```python
from build123d import *

# Parameters (mm, degrees)
SKETCH1_R           = 1.4
BOSS_EXTRUDE1_DEPTH = 19
SKETCH2_R           = 1.7
BOSS_EXTRUDE2_DEPTH = 0.7
FILLET1_R           = 0.5
SKETCH3_R           = 1.7
BOSS_EXTRUDE3_DEPTH = 0.7
FILLET2_R           = 0.5


with BuildPart() as part:
    # Sketch1 → Boss-Extrude1 (new body)
    with BuildSketch(Plane(origin=(0, 0, 0), x_dir=(1, 0, 0), z_dir=(0, 1, 0))):
        Circle(SKETCH1_R)
    extrude(amount=BOSS_EXTRUDE1_DEPTH)

    # Sketch2 → Boss-Extrude2 (add)
    with BuildSketch(Plane(origin=(0, 19, 0), x_dir=(1, 0, 0), z_dir=(0, 1, 0))):
        Circle(SKETCH2_R)
    extrude(amount=BOSS_EXTRUDE2_DEPTH)

    # Fillet1
    fillet1_edges = [part.edges().sort_by_distance(p)[0] for p in [
        (-1.7, 19.7, 0),
    ]]
    fillet(fillet1_edges, radius=FILLET1_R)

    # Sketch3 → Boss-Extrude3 (add)
    with BuildSketch(Plane.XZ):
        Circle(SKETCH3_R)
    extrude(amount=BOSS_EXTRUDE3_DEPTH)

    # Fillet2
    fillet2_edges = [part.edges().sort_by_distance(p)[0] for p in [
        (-1.7, -0.7, 0),
    ]]
    fillet(fillet2_edges, radius=FILLET2_R)


solid = part.part
```
Source: CAD feature listing. Evaluate the final solid. Frame: model axes, mm. Coordinates: 2 decimals unless noted, no trailing zeros. Loops run counter-clockwise (first coordinate to the right, second up) from the corner with the lowest first, then second, coordinate; pieces in that order, holes last. Notation, with made-up numbers: (40.25, 39) -> (44.25, 39) arc R19 cw to (44.25, 54) -> close; hole circle Ø8 at (51.25, 30). An arc over 180 degrees is marked (long way). One line per item, written item: value. Start each with the question number.
Q1. Contact query for flat-ended pins moving along their axis: P1, Ø1.5, axis at y = 9.5, z = 1, coming from the +X side; P2, Ø1, axis at y = 2, z = 1, coming from the -X side; P3, Ø1.5, axis at y = 4.5, z = 0.5, coming from the -X side. Output: stop coordinate, or through.
Q2. Section query A-A, the plane z = 0. Return the cut outline in (x, y).
Q3. Line query: line 1 along X through (y, z) = (6, 0); line 2 along Y through (x, z) = (-0.85, -0.9). Output: solid intervals per line, ascending.
Q4. Section query C-C, the plane y = 14.25. Return the cut outline in (x, z).
Q5. Mould query, pull axis Y, two halves, no side actions, for faces 1 (the face through (0, 19.7, 0)), 2 (the face through (0, -0.7, 0)), 3 (the face through (-1.4, 9.37, -0.06)). Classes: pulls with the +Y half, pulls with the -Y half, needs draft (parallel to the pull), parting line crosses it, or undercut.
Q6. Section query B-B, the plane x = 0. Return the cut outline in (y, z), and give its area (3 significant figures).
Results:
1. P1: x = 1.38
1. P2: x = -1.31
1. P3: x = -1.4
2. outline: (-1.7, -0.2) arc R0.5 ccw to (-1.2, -0.7) -> (1.2, -0.7) arc R0.5 ccw to (1.7, -0.2) -> (1.7, 0) -> (1.4, 0) -> (1.4, 19) -> (1.7, 19) -> (1.7, 19.2) arc R0.5 ccw to (1.2, 19.7) -> (-1.2, 19.7) arc R0.5 ccw to (-1.7, 19.2) -> (-1.7, 19) -> (-1.4, 19) -> (-1.4, 0) -> (-1.7, 0) -> close
3. line 1: -1.4 to 1.4
3. line 2: -0.7 to 19.7
4. outline: circle Ø2.8 at (0, 0)
5. face 1: pulls with the +Y half
5. face 2: pulls with the -Y half
5. face 3: undercut
6. outline: (-0.7, -1.2) arc R0.5 ccw to (-0.2, -1.7) -> (0, -1.7) -> (0, -1.4) -> (19, -1.4) -> (19, -1.7) -> (19.2, -1.7) arc R0.5 ccw to (19.7, -1.2) -> (19.7, 1.2) arc R0.5 ccw to (19.2, 1.7) -> (19, 1.7) -> (19, 1.4) -> (0, 1.4) -> (0, 1.7) -> (-0.2, 1.7) arc R0.5 ccw to (-0.7, 1.2) -> close
6. area: 57.7 mm^2
